```python
from build123d import *

# Parameters (mm, degrees)
CYLINDER003_R     = 12.6
CYLINDER003_DEPTH = 17
BOX_W             = 6.4
BOX_H             = 7.4
BOX_DEPTH         = 10
CYLINDER002_R     = 15.4
CYLINDER002_DEPTH = 3
CYLINDER001_R     = 14.4
CYLINDER001_DEPTH = 12
CYLINDER_R        = 17.4
CYLINDER_DEPTH    = 10
BOX001_W          = 13
BOX001_H          = 13
BOX001_DEPTH      = 5


with BuildPart() as cylinder003:
    # Cylinder003 → Cylinder003 (new body)
    with BuildSketch(Plane(origin=(3.4, 3.4, -6), x_dir=(1, 0, 0), z_dir=(0, 0, 1))):
        Circle(CYLINDER003_R)
    extrude(amount=CYLINDER003_DEPTH)


with BuildPart() as cube:
    # Box → Box (new body)
    with BuildSketch(Plane.XY):
        with Locations((3.2, 3.7)):
            Rectangle(BOX_W, BOX_H)
    extrude(amount=BOX_DEPTH)


with BuildPart() as cylinder002:
    # Cylinder002 → Cylinder002 (new body)
    with BuildSketch(Plane(origin=(3.2, 3.5, 0), x_dir=(1, 0, 0), z_dir=(0, 0, 1))):
        Circle(CYLINDER002_R)
    extrude(amount=CYLINDER002_DEPTH)


with BuildPart() as cylinder001:
    # Cylinder001 → Cylinder001 (new body)
    with BuildSketch(Plane(origin=(3.2, 3.5, 0), x_dir=(1, 0, 0), z_dir=(0, 0, 1))):
        Circle(CYLINDER001_R)
    extrude(amount=CYLINDER001_DEPTH)


with BuildPart() as cut:
    # Cylinder → Cylinder (new body)
    with BuildSketch(Plane(origin=(3.2, 3.5, 0), x_dir=(1, 0, 0), z_dir=(0, 0, 1))):
        Circle(CYLINDER_R)
    extrude(amount=CYLINDER_DEPTH)

    # Cut: cut Cylinder001
    add(cylinder001.part, mode=Mode.SUBTRACT)


with BuildPart() as common:
    # Box001 → Box001 (new body)
    with BuildSketch(Plane(origin=(-3.4, -2.8, 0), x_dir=(1, 0, 0), z_dir=(0, 0, 1))):
        with Locations((6.5, 6.5)):
            Rectangle(BOX001_W, BOX001_H)
    extrude(amount=BOX001_DEPTH)

    # Fusion: union Cylinder002, Cut
    add(cylinder002.part)
    add(cut.part)

    # Cut001: cut Cube
    add(cube.part, mode=Mode.SUBTRACT)

    # Common: intersect Cylinder003
    add(cylinder003.part, mode=Mode.INTERSECT)


solid = common.part
```
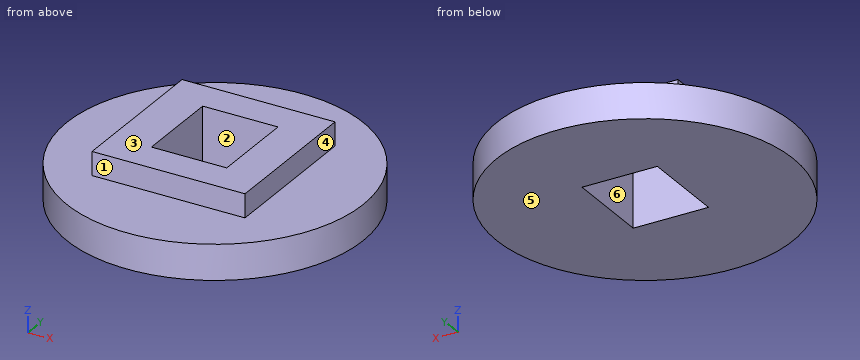
Model file for the job. Use its own axes, mm. Face numbers are marked on the shaded views. A direction names the side the tool comes from. Round coordinates to 2 decimals unless told otherwise and drop trailing zeros. Loops run counter-clockwise (first coordinate to the right, second up) from the corner with the lowest first, then second, coordinate; pieces in that order, holes last. Notation, with made-up numbers: M 37,-10.5 L 53,-10.5 A20 cw 53,11.5 Z; hole C 54,49 d5. An arc over 180 degrees is marked long. Put each result on its own line as item: value. Start each with the question number.
Item 1: Mould opens along Y. For the marked faces 1, 2 and 3 say: released by +Y, released by -Y, zero draft, split by the parting line, or undercut.
Item 2: 3-axis set-ups, long thin cutter, end or side, ignore diameter. For the marked faces 4, 5 and 6: which of +Z, -Z, +X, -X, +Y, -Y reach the whole face in a straight line?
Item 3: Cut at D-D (z = 1.9). List the corners of the cut face in (x, y).
Item 4: Cut at C-C (z = 3.9). List the corners of the cut face in (x, y).
Item 5: Cut at B-B (y = 3.4). List the corners of the cut face in (x, z).
Item 6: Drop flat-ended pins along their axis: P1, Ø0.6, axis at x = 2.5, z = 4, coming from the +Y side; P2, Ø2, axis at x = -1.5, z = 3.5, coming from the +Y side; P3, Ø1.5, axis at x = 1.5, z = 2, coming from the +Y side. Give the stop position or say it passes through.
Item 7: Drill centre lines: line 1 along X through (y, z) = (3, 3.15); line 2 along Y through (x, z) = (2.25, 4.3); line 3 along Z through (x, y) = (14.75, 2.5). Where is each one in solid material? Low to high.
Item 8: Cut at A-A (x = 3.4). List the corners of the cut face in (y, z).
Answer block:
1. face 1: released by -Y
1. face 2: undercut
1. face 3: zero draft
2. face 4: +Z, +X, +Y, -Y
2. face 5: -Z, +X, -X, +Y, -Y
2. face 6: +Z, -Z
3. outline: C 3.4,3.4 d25.2; hole M 0,0 L 6.4,0 L 6.4,7.4 L 0,7.4 Z
4. outline: M -3.4,-2.8 L 9.6,-2.8 L 9.6,10.2 L -3.4,10.2 Z; hole M 0,0 L 6.4,0 L 6.4,7.4 L 0,7.4 Z
5. outline: M -9.2,0 L 0,0 L 0,5 L -3.4,5 L -3.4,3 L -9.2,3 Z; M 6.4,0 L 16,0 L 16,3 L 9.6,3 L 9.6,5 L 6.4,5 Z
6. P1: y = 10.2
6. P2: y = 15.34
6. P3: y = 15.95
7. line 1: -3.4 to 0, 6.4 to 9.6
7. line 2: -2.8 to 0, 7.4 to 10.2
7. line 3: 0 to 3
8. outline: M -9.2,0 L 0,0 L 0,5 L -2.8,5 L -2.8,3 L -9.2,3 Z; M 7.4,0 L 16,0 L 16,3 L 10.2,3 L 10.2,5 L 7.4,5 Z
